from build123d import *

# Parameters (mm, degrees)
SKETCH1_W           = 228.6
SKETCH1_H           = 215.9
BOSS_EXTRUDE1_DEPTH = 5.334
SKETCH8_W           = 25.4
SKETCH8_H           = 5.334
CUT_EXTRUDE2_DEPTH  = 6.334
SKETCH11_R          = 1.524
CUT_EXTRUDE4_DEPTH  = 6.334
CUT_EXTRUDE5_DEPTH  = 6.334
CUT_EXTRUDE6_DEPTH  = 6.334
CIRPATTERN1_COUNT   = 8
CUT_EXTRUDE7_DEPTH  = 6.334


with BuildPart() as part:
    # Sketch1 → Boss-Extrude1 (new body)
    with BuildSketch(Plane(origin=(0, 0, 0), x_dir=(1, 0, 0), z_dir=(0, 1, 0))):
        with Locations((114.3, 107.95)):
            Rectangle(SKETCH1_W, SKETCH1_H)
    extrude(amount=BOSS_EXTRUDE1_DEPTH)

    # Sketch8 → Cut-Extrude2 (cut, through all)
    with BuildSketch(Plane(origin=(0, 5.334, 0), x_dir=(1, 0, 0), z_dir=(0, 1, 0))):
        with Locations((18.034, 131.826)):
            Rectangle(SKETCH8_W, SKETCH8_H)
        with Locations((210.566, 131.826)):
            Rectangle(SKETCH8_W, SKETCH8_H)
        with Locations((210.566, 84.074)):
            Rectangle(SKETCH8_W, SKETCH8_H)
        with Locations((18.034, 84.074)):
            Rectangle(SKETCH8_W, SKETCH8_H)
    extrude(amount=-CUT_EXTRUDE2_DEPTH, mode=Mode.SUBTRACT)

    # Sketch11 → Cut-Extrude4 (cut, through all)
    with BuildSketch(Plane(origin=(0, 5.334, 0), x_dir=(1, 0, 0), z_dir=(0, 1, 0))):
        with Locations((95.758, 6.604)):
            Circle(SKETCH11_R)
        with Locations((132.842, 6.604)):
            Circle(SKETCH11_R)
        with Locations((132.842, 43.688)):
            Circle(SKETCH11_R)
        with Locations((95.758, 43.688)):
            Circle(SKETCH11_R)
    extrude(amount=-CUT_EXTRUDE4_DEPTH, mode=Mode.SUBTRACT)

    # Sketch13 → Cut-Extrude5 (cut, through all)
    with BuildSketch(Plane(origin=(0, 5.334, 0), x_dir=(1, 0, 0), z_dir=(0, 1, 0))):
        Polygon((0, 215.9), (0, 161.925), (57.15, 215.9), align=None)
        Polygon((228.6, 161.925), (171.45, 215.9), (228.6, 215.9), align=None)
        Polygon((228.6, 0), (228.6, 53.975), (171.45, 0), align=None)
        Polygon((0, 53.975), (57.15, 0), (0, 0), align=None)
    extrude(amount=-CUT_EXTRUDE5_DEPTH, mode=Mode.SUBTRACT)

    # Sketch6 → Cut-Extrude6 (cut, through all)
    with BuildSketch(Plane(origin=(0, 5.334, 0), x_dir=(1, 0, 0), z_dir=(0, 1, 0))):
        with BuildLine():
            Line((114.3, 165.1), (114.3, 160.02))
            ThreePointArc((114.3, 160.02), (124.427414599, 159.025633853), (134.168028422, 156.080513675))
            ThreePointArc((134.168028422, 156.080513675), (134.197181023, 156.068469295), (134.226326323, 156.056407258))
            Line((134.226326323, 156.056407258), (136.17035816, 160.749715283))
            ThreePointArc((136.17035816, 160.749715283), (125.449411903, 164.001878775), (114.3, 165.1))
        make_face()
    cut_extrude6 = extrude(amount=-CUT_EXTRUDE6_DEPTH, mode=Mode.SUBTRACT)

    # CirPattern1: Cut-Extrude6 ×8 about axis
    cirpattern1_axis = Axis((114.3, 0, -107.95), (0, 1, 0))
    for i in range(1, CIRPATTERN1_COUNT):
        add(cut_extrude6.rotate(cirpattern1_axis, i * 360 / CIRPATTERN1_COUNT), mode=Mode.SUBTRACT)

    # Sketch16 → Cut-Extrude7 (cut, through all)
    with BuildSketch(Plane(origin=(0, 5.334, 0), x_dir=(1, 0, 0), z_dir=(0, 1, 0))):
        Polygon((180.893807675, 189.512113449), (199.35994175, 172.071875712), (195.697491825, 168.193987556), (177.23135775, 185.634225293), align=None)
        Polygon((47.706192325, 189.512113449), (51.36864225, 185.634225293), (32.902508175, 168.193987556), (29.24005825, 172.071875712), align=None)
        Polygon((47.706192325, 26.387886551), (29.24005825, 43.828124288), (32.902508175, 47.706012444), (51.36864225, 30.265774707), align=None)
        Polygon((180.893807675, 26.387886551), (177.23135775, 30.265774707), (195.697491825, 47.706012444), (199.35994175, 43.828124288), align=None)
    extrude(amount=-CUT_EXTRUDE7_DEPTH, mode=Mode.SUBTRACT)


solid = part.part
Check sheet for the modelled part. Datum: model origin and axes. Units: mm. A direction names the side the tool comes from. Round coordinates to 2 decimals unless told otherwise and drop trailing zeros. Loops run counter-clockwise (first coordinate to the right, second up) from the corner with the lowest first, then second, coordinate; pieces in that order, holes last. Notation, with made-up numbers: (-11, 67.5) -> (12, 67.5) arc R30 ccw to (12, 95.5) -> close; hole circle Ø4 at (83.25, 58). An arc over 180 degrees is marked (long way). Put each result on its own line as item: value. Start each with the question number.
1. Section check C-C (x = 17). Enter the section's corners in (y, z), plus the area to 3 significant figures.
2. Section check B-B (x = 128). Enter the section's corners in (y, z), plus the area to 3 significant figures.
3. Access from +Z, -Z, +X, -X, +Y, -Y to the whole of each face (thin tool, end or side, straight path). Record for faces 1 (the face through (0, 3, -107)), 2 (the face through (125.6, 2.7, -163.97)).
4. Draft check along Z on faces 3 (the face through (113, 5.334, -109)), 4 (the face through (200.43, 2.7, -27.37)), 5 (the face through (18, 3, -129.159)). Enter one of: +Z half, -Z half, draft (parallel to the pull), parting line (faces both ways), or undercut.
5. Scan lines: probe 1 along X at (y, z) = (4.35, -179.5); probe 2 along Z at (x, y) = (29, 4.65); probe 3 along Z at (x, y) = (204, 3.5). Record each from-to range of solid material in increasing order.
6. Gauge pin test, flat ends, axial feed: pin 1 (2.5 mm diameter, centred on x = 12, y = 2, fed in from -Z); pin 2 (2.5 mm diameter, centred on x = 132.842, z = -43.688, fed in from -Y); pin 3 (2.5 mm diameter, centred on x = 216, y = 3, fed in from +Z); pin 4 (1.5 mm diameter, centred on x = 179.5, y = 3.5, fed in from +Z). Record the tip position at first contact, or that the pin passes through.
7. Section check D-D (z = -33.5). Enter the section's corners in (x, y), plus the area to 3 significant figures.
8. Section check A-A (z = -99). Enter the section's corners in (x, y).
Findings:
1. outline: (0, -177.98) -> (5.33, -177.98) -> (5.33, -134.49) -> (0, -134.49) -> close; (0, -129.16) -> (5.33, -129.16) -> (5.33, -86.74) -> (0, -86.74) -> close; (0, -81.41) -> (5.33, -81.41) -> (5.33, -37.92) -> (0, -37.92) -> close
1. area: 690 mm^2
2. outline: (0, -215.9) -> (5.33, -215.9) -> (5.33, -163.43) -> (0, -163.43) -> close; (0, -158.19) -> (5.33, -158.19) -> (5.33, 0) -> (0, 0) -> close
2. area: 1,120 mm^2
3. face 1: +Z, -Z, -X, +Y, -Y
3. face 2: +Y, -Y
4. face 3: draft
4. face 4: +Z half
4. face 5: undercut
5. probe 1: x = 18.61 to 37.11, 44.87 to 183.73, 191.49 to 209.99
5. probe 2: z = -189.31 to -134.49, -129.16 to -86.74, -81.41 to -26.59
5. probe 3: z = -185.16 to -134.49, -129.16 to -86.74, -81.41 to -30.74
6. pin 1: stops at z = -174.44
6. pin 2: passes through
6. pin 3: stops at z = -40.89
6. pin 4: stops at z = -6.89
7. outline: (21.68, 0) -> (40.18, 0) -> (40.18, 5.33) -> (21.68, 5.33) -> close; (47.94, 0) -> (180.66, 0) -> (180.66, 5.33) -> (47.94, 5.33) -> close; (188.42, 0) -> (206.92, 0) -> (206.92, 5.33) -> (188.42, 5.33) -> close
7. area: 905 mm^2
8. outline: (0, 0) -> (165.6, 0) -> (165.6, 5.33) -> (0, 5.33) -> close; (170.74, 0) -> (228.6, 0) -> (228.6, 5.33) -> (170.74, 5.33) -> close
